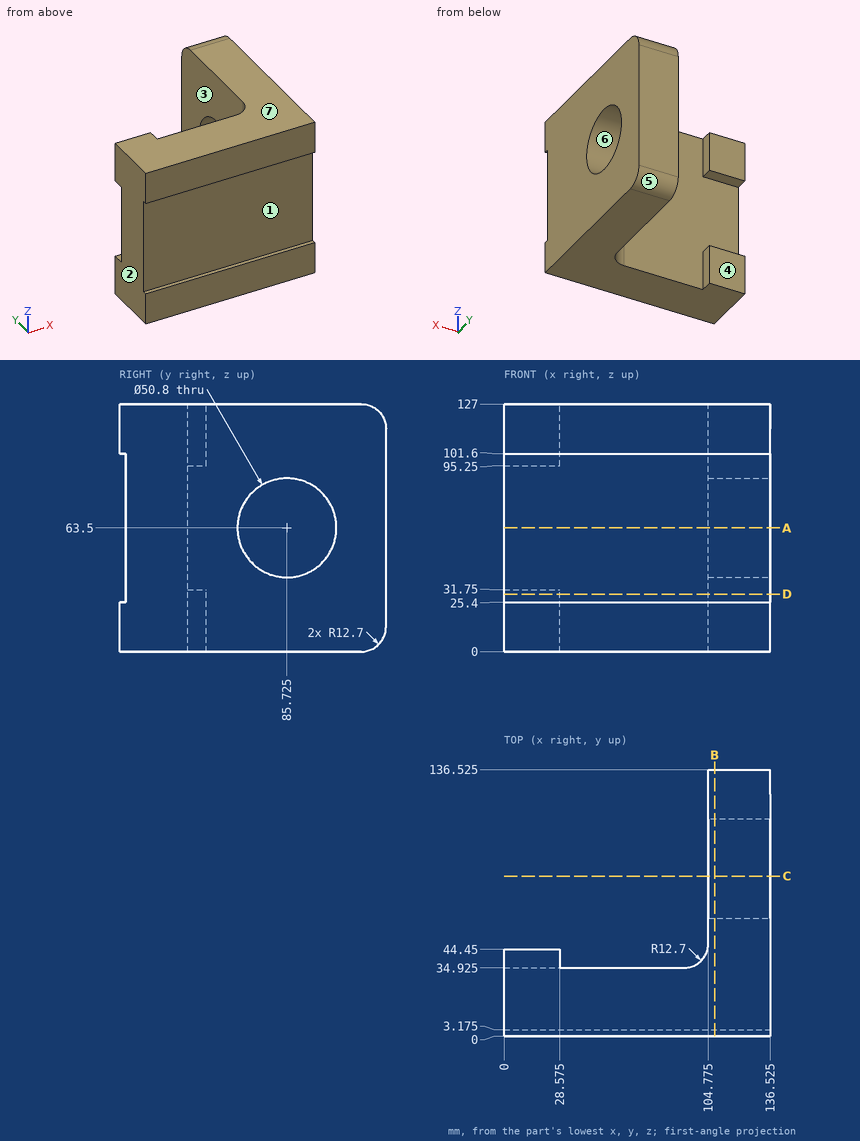
Geometry: see drawing. Coordinates: mm, zero at the bounding-box minimum. A direction names the side the tool comes from. Give positions to 0.01 mm unless a question says otherwise; leave off trailing zeros. Order: outer loops, then holes, each group sorted by start corner. A loop starts at its lowest first (then second) coordinate and runs counter-clockwise, first axis right, second up. Notation, with made-up numbers: (27.5, -14) -> (80.5, -14) arc R18 ccw to (80.5, 9) -> close; hole circle Ø8 at (-23, 65.5). An arc over 180 degrees is marked (long way). Write each question's results on one line, items separated by ' | '.
1) Line query: line 1 along X through (y, z) = (103.5, 92) (3 decimals); line 2 along X through (y, z) = (44, 17) (3 decimals); line 3 along Y through (x, z) = (57, 15) (3 decimals). Output: solid intervals per line, ascending.
Geometry says:
line 1: x = 104.775 to 136.525 | line 2: x = 0 to 28.575, 104.247 to 136.525 | line 3: y = 0 to 34.925
2) Cut plane A-A (z = 63.5). Output: boundary loops of the cut face in (x, y) (3 decimals), and give its area (3 significant figures).
Geometry says:
outline: (0, 3.175) -> (136.525, 3.175) -> (136.525, 60.325) -> (104.775, 60.325) -> (104.775, 47.625) arc R12.7 cw to (92.075, 34.925) -> (0, 34.925) -> close; (104.775, 111.125) -> (136.525, 111.125) -> (136.525, 136.525) -> (104.775, 136.525) -> close | area: 5,980 mm²
3) Cut plane B-B (x = 108). Output: boundary loops of the cut face in (y, z) (3 decimals), and give its area (3 significant figures).
Geometry says:
outline: (0, 0) -> (123.825, 0) arc R12.7 ccw to (136.525, 12.7) -> (136.525, 114.3) arc R12.7 ccw to (123.825, 127) -> (0, 127) -> (0, 101.6) -> (3.175, 101.6) -> (3.175, 25.4) -> (0, 25.4) -> close; hole circle Ø50.8 at (85.725, 63.5) | area: 15,000 mm²
4) Set-up query: the marked faces 1, 2 and 3. Return all of +Z, -Z, +X, -X, +Y, -Y with unobstructed straight access to the full face (end or side cutting, diameter ignored); none if empty.
Geometry says:
face 1: +X, -X, -Y | face 2: +Z, -Z, -X, +Y, -Y | face 3: +Z, -Z, -X, +Y
5) Draft query along Z for the marked faces 4, 5, 6 and 7. Return one class per face: released by +Z, released by -Z, zero draft, split by the parting line, or undercut.
Geometry says:
face 4: zero draft | face 5: released by -Z | face 6: undercut | face 7: released by +Z
6) Cut plane D-D (z = 29.5). Output: boundary loops of the cut face in (x, y) (3 decimals).
Geometry says:
outline: (0, 3.175) -> (136.525, 3.175) -> (136.525, 136.525) -> (104.775, 136.525) -> (104.775, 47.625) arc R12.7 cw to (92.075, 34.925) -> (28.575, 34.925) -> (28.575, 44.45) -> (0, 44.45) -> close
7) First-contact query: pin 1 Ø14.5 at (x, z) = (16, 13) entering from +Y; pin 2 Ø4 at (x, z) = (74.5, 78) entering from -Y (3 decimals); pin 3 Ø1.5 at (x, z) = (55.5, 26) entering from +Y (3 decimals). Flat tips, straight axial feed; report the tip coordinate or a pass-through.
Geometry says:
pin 1: stops at y = 44.45 | pin 2: stops at y = 3.175 | pin 3: stops at y = 34.925
8) Cut plane C-C (y = 82). Output: boundary loops of the cut face in (x, z) (3 decimals), and give its area (3 significant figures).
Geometry says:
outline: (104.775, 0) -> (136.525, 0) -> (136.525, 38.375) -> (104.775, 38.375) -> close; (104.775, 88.625) -> (136.525, 88.625) -> (136.525, 127) -> (104.775, 127) -> close | area: 2,440 mm²
